```python
from build123d import *

# Parameters (mm, degrees)
RESSALTO_EXTRUS_O1_DEPTH = 15
ESBO_O3_R                = 2.5
CORTE_EXTRUS_O1_DEPTH    = 15
CHANFRO1_SIZE            = 2
FILETE1_R                = 0.5
CHANFRO5_SIZE            = 2
CHANFRO7_SIZE            = 5
CHANFRO9_SIZE            = 1
CORTE_EXTRUS_O2_DEPTH    = 5


with BuildPart() as part:
    # Esboço1 → Ressalto-extrusão1 (new body)
    with BuildSketch(Plane.XY):
        Polygon((0.299414955, -0.75), (-5.700585045, -0.75), (-5.700585045, -17.25), (14.299414955, -17.25), (14.299414955, -22.25), (-10.700585045, -22.25), (-10.700585045, -0.75), (-110.700585045, -0.75), (-110.700585045, 4.25), (0.299414955, 4.25), align=None)
    extrude(amount=RESSALTO_EXTRUS_O1_DEPTH)

    # Esboço3 → Corte-extrusão1 (cut)
    with BuildSketch(Plane.XZ.offset(22.25)):
        with Locations(Location((6.299414955, 7.5, 0), (0, 0, 270))):
            Circle(ESBO_O3_R)
    extrude(amount=-CORTE_EXTRUS_O1_DEPTH, mode=Mode.SUBTRACT)

    # Chanfro1
    chanfro1_edges = [part.edges().sort_by_distance(p)[0] for p in [
        (6.299414955, -22.25, 10),
    ]]
    chamfer(chanfro1_edges, length=CHANFRO1_SIZE)

    # Filete1
    filete1_edges = [part.edges().sort_by_distance(p)[0] for p in [
        (6.299414955, -17.25, 10),
    ]]
    fillet(filete1_edges, radius=FILETE1_R)

    # Chanfro5
    chanfro5_edges = [part.edges().sort_by_distance(p)[0] for p in [
        (14.299414955, -22.25, 7.5),
        (-10.700585045, -22.25, 7.5),
        (0.299414955, 4.25, 7.5),
    ]]
    chamfer(chanfro5_edges, length=CHANFRO5_SIZE)

    # Chanfro7
    chanfro7_edges = [part.edges().sort_by_distance(p)[0] for p in [
        (-10.700585045, -0.75, 7.5),
    ]]
    chamfer(chanfro7_edges, length=CHANFRO7_SIZE)

    # Chanfro9
    chanfro9_edges = [part.edges().sort_by_distance(p)[0] for p in [
        (13.299414955, -21.25, 0),
        (14.299414955, -18.75, 0),
        (0.299414955, 0.75, 0),
        (-0.700585045, 3.25, 0),
        (-56.200585045, 4.25, 0),
        (-110.700585045, 1.75, 0),
        (-63.200585045, -0.75, 0),
        (-13.200585045, -3.25, 0),
        (-10.700585045, -13, 0),
        (-9.700585045, -21.25, 0),
        (1.799414955, -22.25, 0),
        (-110.700585045, 1.75, 15),
        (-56.200585045, 4.25, 15),
        (-0.700585045, 3.25, 15),
        (0.299414955, 0.75, 15),
        (14.299414955, -18.75, 15),
        (13.299414955, -21.25, 15),
        (1.799414955, -22.25, 15),
        (-9.700585045, -21.25, 15),
        (-10.700585045, -13, 15),
        (-13.200585045, -3.25, 15),
        (-63.200585045, -0.75, 15),
        (-110.700585045, 4.25, 7.5),
        (-110.700585045, -0.75, 7.5),
    ]]
    chamfer(chanfro9_edges, length=CHANFRO9_SIZE)

    # Esboço4 → Corte-extrusão2 (cut)
    with BuildSketch(Plane(origin=(0, -10.75, 0), x_dir=(1, 0, 0), z_dir=(0, 0, -1))):
        with BuildLine():
            Line((-104.993478264, -11.6), (-19.993478264, -11.6))
            ThreePointArc((-19.993478264, -11.6), (-19.093478264, -12.5), (-19.993478264, -13.4))
            Line((-19.993478264, -13.4), (-104.993478264, -13.4))
            ThreePointArc((-104.993478264, -13.4), (-105.893478264, -12.5), (-104.993478264, -11.6))
        make_face()
    extrude(amount=-CORTE_EXTRUS_O2_DEPTH, mode=Mode.SUBTRACT)


solid = part.part
```
Geometry check sheet. Reference: the model listing, model coordinates, mm. A direction names the side the tool comes from. Give positions to 0.01 mm unless a question says otherwise; leave off trailing zeros. Write each loop counter-clockwise with the first axis right and the second up, starting at its lowest first coordinate (ties: lowest second). Pieces come first, ordered by that corner, then holes. Notation, with made-up numbers: (15, -30) - (60, -30) arc R24 cw to (60, -9) - close; hole circle Ø1 at (20.5, 39). An arc over 180 degrees is marked (long way). Use a Markdown table: item, result.
Q1. Go/stop test with flat-tipped pins: P1, Ø1.5, axis at x = -56.5, z = 1.5, coming from the -Y side; P2, Ø1.5, axis at x = -30, z = 9, coming from the -Y side; P3, Ø7.5, axis at x = 3.5, z = 8.5, coming from the +Y side. Record where each tip stops, or that it passes through.
Computed:
| item | result |
|---|---|
| P1 | stops at y = -0.75 |
| P2 | stops at y = -0.75 |
| P3 | stops at y = 2.8 |
Q2. Section check B-B, the plane x = -17. Enter the section's corners in (y, z), then the cut area to 3 significant figures.
Computed:
| item | result |
|---|---|
| outline | (-0.75, 1) - (0.25, 0) - (3.25, 0) - (4.25, 1) - (4.25, 14) - (3.25, 15) - (0.25, 15) - (-0.75, 14) - close |
| area | 73.0 mm² |
Q3. Section check C-C, the plane y = -10.75. Enter the section's corners in (x, z).
Computed:
| item | result |
|---|---|
| outline | (-10.7, 1) - (-9.7, 0) - (-5.7, 0) - (-5.7, 15) - (-9.7, 15) - (-10.7, 14) - close |
Q4. Draft check along X on faces 1 (the face through (-10.701, -13, 7)), 2 (the face through (-1.073, 2.905, 14.507)), 3 (the face through (-63, 0.85, 2)), 4 (the face through (3.86, -19.02, 8.04)). Enter one of: pulls with the +X half, pulls with the -X half, needs draft (parallel to the pull), parting line crosses it, or undercut.
Computed:
| item | result |
|---|---|
| face 1 | pulls with the -X half |
| face 2 | pulls with the +X half |
| face 3 | undercut |
| face 4 | undercut |
Q5. Set-up check for faces 5 (the face through (-9.71, -21.24, 7.41)), 6 (the face through (-3, -0.75, 7)), 7 (the face through (0.299, 1, 7)): record each of +Z, -Z, +X, -X, +Y, -Y from which the full face is reachable in a straight line by a thin tool's end or side.
Computed:
| item | result |
|---|---|
| face 5 | +Z, -Z, -X, -Y |
| face 6 | +Z, -Z, +X |
| face 7 | +Z, -Z, +X, +Y |
Q6. Section check D-D, the plane x = -68. Enter the section's corners in (y, z), then the cut area to 3 significant figures.
Computed:
| item | result |
|---|---|
| outline | (-0.75, 1) - (0.25, 0) - (0.85, 0) - (0.85, 5) - (2.65, 5) - (2.65, 0) - (3.25, 0) - (4.25, 1) - (4.25, 14) - (3.25, 15) - (0.25, 15) - (-0.75, 14) - close |
| area | 64.0 mm² |
Q7. Thickness scan on L1, parallel to X at y = -19.3, z = 7.5; L2, parallel to Y at x = -70, z = 3.25; L3, parallel to Y at x = -64.5, z = 8.5. Record the ranges inside material, lowest first. Write a range as [from, to].
Computed:
| item | result |
|---|---|
| L1 | x = [-10.7, 3.8], [8.8, 14.3] |
| L2 | y = [-0.75, 0.85], [2.65, 4.25] |
| L3 | y = [-0.75, 4.25] |
Q8. Section check A-A, the plane z = 7.5. Enter the section's corners in (x, y).
Computed:
| item | result |
|---|---|
| outline | (-110.7, 0.25) - (-109.7, -0.75) - (-15.7, -0.75) - (-10.7, -5.75) - (-10.7, -20.25) - (-8.7, -22.25) - (1.8, -22.25) - (3.8, -20.25) - (3.8, -17.75) arc R0.5 ccw to (3.3, -17.25) - (-5.7, -17.25) - (-5.7, -0.75) - (0.3, -0.75) - (0.3, 2.25) - (-1.7, 4.25) - (-109.7, 4.25) - (-110.7, 3.25) - close; (8.8, -20.25) - (10.8, -22.25) - (12.3, -22.25) - (14.3, -20.25) - (14.3, -17.25) - (9.3, -17.25) arc R0.5 ccw to (8.8, -17.75) - close |
